from build123d import *

# Parameters (mm, degrees)
BOSS_EXTRU_1_DEPTH = 0.5
BOSS_EXTRU_2_DEPTH = 1.5


with BuildPart() as part:
    # Esquisse1 → Boss.-Extru.1 (new body)
    with BuildSketch(Plane.XY):
        with BuildLine():
            Line((0, -2), (80, -2))
            ThreePointArc((80, -2), (82, 0), (80, 2))
            Line((80, 2), (0, 2))
            ThreePointArc((0, 2), (-2, 0), (0, -2))
        make_face()
    extrude(amount=BOSS_EXTRU_1_DEPTH)

    # Esquisse2 → Boss.-Extru.2 (add)
    with BuildSketch(Plane.XY.offset(0.5)):
        with BuildLine():
            Line((-0.809863383, -1.164625511), (1.809863383, -1.164625511))
            Line((1.809863383, -1.164625511), (1.809863383, 1.164625511))
            Line((1.809863383, 1.164625511), (-0.809863383, 1.164625511))
            ThreePointArc((-0.809863383, 1.164625511), (-1.516970164, 0.871732292), (-1.809863383, 0.164625511))
            Line((-1.809863383, 0.164625511), (-1.809863383, -0.164625511))
            ThreePointArc((-1.809863383, -0.164625511), (-1.516970164, -0.871732292), (-0.809863383, -1.164625511))
        make_face()
    extrude(amount=BOSS_EXTRU_2_DEPTH)


solid = part.part
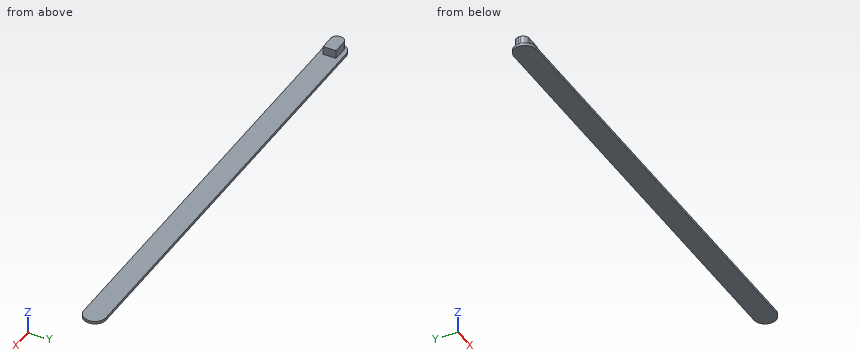
The listing builds one solid part. Answer for the finished solid, in the listing's coordinates (mm). Round coordinates to 2 decimals unless told otherwise and drop trailing zeros. Write each loop counter-clockwise with the first axis right and the second up, starting at its lowest first coordinate (ties: lowest second). Pieces come first, ordered by that corner, then holes. Notation, with made-up numbers: M 17,64.25 L 26,64.25 A23 cw 26,74.25 Z; hole C 3,39.25 d4. An arc over 180 degrees is marked long. Write each question's results on one line, items separated by ' | '. Start each with the question number.
(1) The part is cut by section B-B, the plane x = 18.5. Write down the section's boundary in (y, z), and give its area (3 significant figures).
(2) The part is cut by section A-A, the plane z = 0.8. Write down the section's boundary in (x, y).
(3) Find the intervals of material crossed by line 1 (Z direction, x = 53, y = 0.85); line 2 (X direction, y = -0.35, z = 0.6); line 3 (X direction, y = 0.25, z = 0.2), in increasing order.
(4) Each of these flat-tipped pins is pushed along its axis until it touches: P1, Ø1.2, axis at x = 45.5, y = 0.5, coming from the +Z side; P2, Ø1.2, axis at x = 0.5, z = 1.5, coming from the +Y side. Where does it stop, or does it pass through?
Worked answers:
1) outline: M -2,0 L 2,0 L 2,0.5 L -2,0.5 Z | area: 2.00 mm²
2) outline: M -1.81,-0.16 A1 ccw -0.81,-1.16 L 1.81,-1.16 L 1.81,1.16 L -0.81,1.16 A1 ccw -1.81,0.16 Z
3) line 1: z = 0 to 0.5 | line 2: x = -1.79 to 1.81 | line 3: x = -1.98 to 81.98
4) P1: stops at z = 0.5 | P2: stops at y = 1.16
